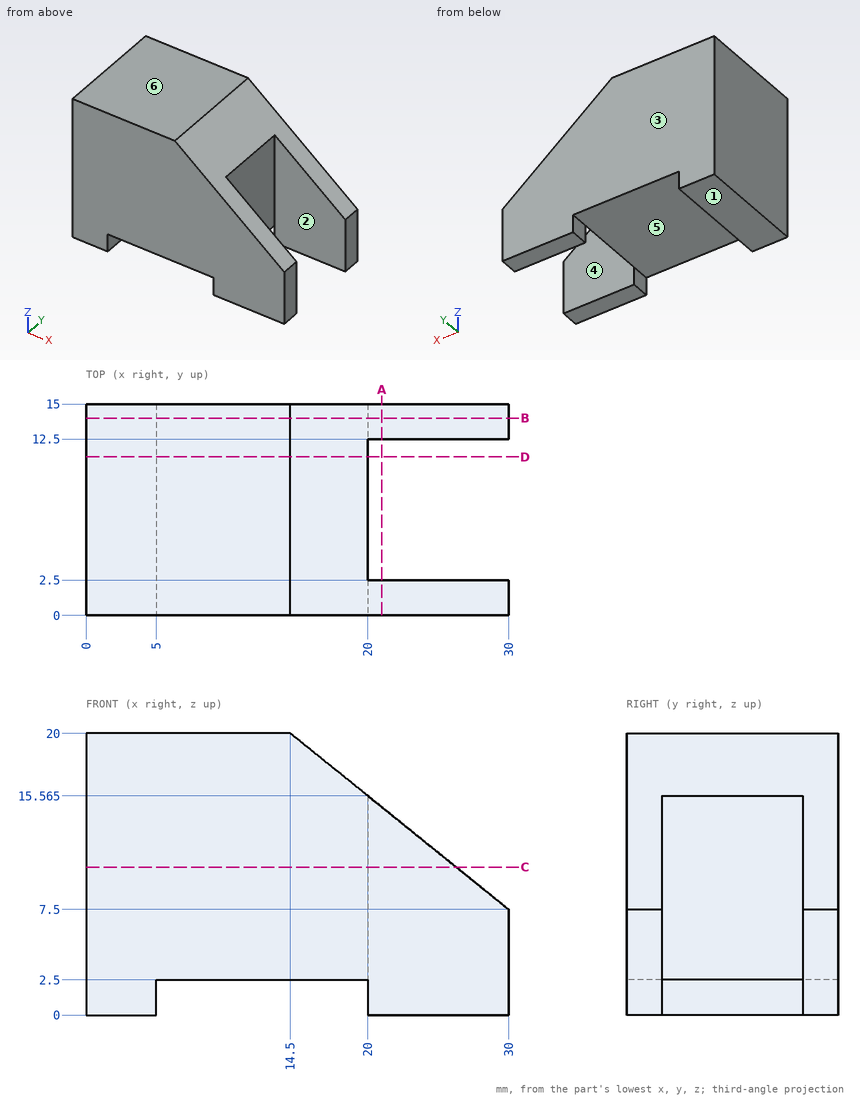
The drawing under review shows one solid part. Ordinate dimensions are in mm from its lowest x, y, z. A direction names the side the tool comes from. Coordinates: 2 decimals unless noted, no trailing zeros. Loops run counter-clockwise (first coordinate to the right, second up) from the corner with the lowest first, then second, coordinate; pieces in that order, holes last.
Item 1: Clearance check with flat-ended pins moving along their axes: pin 1 (5 mm diameter, centred on y = 7, z = 10.5, fed in from +X); pin 2 (0.8 mm diameter, centred on y = 1, z = 1, fed in from -X); pin 3 (4.5 mm diameter, centred on x = 16, y = 8.5, fed in from -Z). State where each tip first meets the part, or that it passes through.
Completed:
pin 1: stops at x = 20
pin 2: stops at x = 0
pin 3: stops at z = 2.5
Item 2: Wall thickness on L1, parallel to Y at x = 20.5, z = 6.5; L2, parallel to Z at x = 13, y = 8; L3, parallel to X at y = 3.5, z = 3.25: over which ranges is each line inside the solid? List them lowest first.
Completed:
L1: y = 0 to 2.5, 12.5 to 15
L2: z = 2.5 to 20
L3: x = 0 to 20
Item 3: Add section A-A (x = 21). Write out the cut boundary in (y, z).
Completed:
outline: (0, 0) - (2.5, 0) - (2.5, 14.76) - (0, 14.76) - close; (12.5, 0) - (15, 0) - (15, 14.76) - (12.5, 14.76) - close
Item 4: For the marked faces 4, 5 and 6, list the 3-axis set-ups (+Z, -Z, +X, -X, +Y, -Y) from which the entire face can be reached by the end or side of a thin tool; tool diameter is ignored.
Completed:
face 4: +Z, -Z, +X
face 5: -Z, +Y, -Y
face 6: +Z, +X, -X, +Y, -Y
Item 5: Add section D-D (y = 11.25). Write out the cut boundary in (x, z) (1 decimal).
Completed:
outline: (0, 0) - (5, 0) - (5, 2.5) - (20, 2.5) - (20, 15.6) - (14.5, 20) - (0, 20) - close
Item 6: Draft analysis for pull direction Y (two halves, no side actions). For the marked faces 1, 2 and 3, state which applies: pulls with the +Y half, pulls with the -Y half, needs draft (parallel to the pull), parting line crosses it, or undercut.
Completed:
face 1: needs draft
face 2: undercut
face 3: pulls with the +Y half
Item 7: Add section B-B (y = 14). Write out the cut boundary in (x, z).
Completed:
outline: (0, 0) - (5, 0) - (5, 2.5) - (20, 2.5) - (20, 0) - (30, 0) - (30, 7.5) - (14.5, 20) - (0, 20) - close
Item 8: Add section C-C (z = 10.5). Write out the cut boundary in (x, y).
Completed:
outline: (0, 0) - (26.28, 0) - (26.28, 2.5) - (20, 2.5) - (20, 12.5) - (26.28, 12.5) - (26.28, 15) - (0, 15) - close
